Source: CAD feature listing. Evaluate the final solid. Frame: model axes, mm. A direction names the side the tool comes from. Round coordinates to 2 decimals unless told otherwise and drop trailing zeros. Write each loop counter-clockwise with the first axis right and the second up, starting at its lowest first coordinate (ties: lowest second). Pieces come first, ordered by that corner, then holes. Notation, with made-up numbers: (52, -32.75) -> (104, -32.75) arc R19 ccw to (104, -28.75) -> close; hole circle Ø11 at (35.5, 17). An arc over 180 degrees is marked (long way). Return JSON: item names as keys, results as strings. Group by question number.
from build123d import *

# Parameters (mm, degrees)
F1_DEPTH = 25
F2_R     = 14.710465
F3_DEPTH = 123


with BuildPart() as f1:
    # F0 (on Front) → F1 (new body)
    with BuildSketch(Plane.XZ):
        with BuildLine():
            ThreePointArc((34.69864, -4.583055), (34.924579, -2.296476), (35, 0))
            ThreePointArc((35, 0), (34.99986, 0.099012), (34.99944, 0.198024))
            ThreePointArc((34.99944, 0.198024), (34.930935, 2.197668), (34.748278, 4.190131))
            ThreePointArc((34.748278, 4.190131), (34.380054, 6.558346), (33.850622, 8.895809))
            ThreePointArc((33.850622, 8.895809), (33.286978, 10.815595), (32.614554, 12.700035))
            ThreePointArc((32.614554, 12.700035), (31.668947, 14.902275), (30.574844, 17.034638))
            ThreePointArc((30.574844, 17.034638), (29.551477, 18.753938), (28.431537, 20.41195))
            ThreePointArc((28.431537, 20.41195), (26.967963, 22.30984), (25.377937, 24.103118))
            ThreePointArc((25.377937, 24.103118), (23.959149, 25.513902), (22.462062, 26.841307))
            ThreePointArc((22.462062, 26.841307), (20.572484, 28.315595), (18.586441, 29.657111))
            ThreePointArc((18.586441, 29.657111), (16.861379, 30.670734), (15.081214, 31.584126))
            ThreePointArc((15.081214, 31.584126), (12.884359, 32.542177), (10.62709, 33.347638))
            ThreePointArc((10.62709, 33.347638), (8.704146, 33.900411), (6.752757, 34.342398))
            ThreePointArc((6.752757, 34.342398), (4.386663, 34.724015), (2, 34.94281))
            ThreePointArc((2, 34.94281), (0, 35), (-2, 34.94281))
            ThreePointArc((-2, 34.94281), (-4.386663, 34.724015), (-6.752757, 34.342398))
            ThreePointArc((-6.752757, 34.342398), (-8.704146, 33.900411), (-10.62709, 33.347638))
            ThreePointArc((-10.62709, 33.347638), (-12.884359, 32.542177), (-15.081214, 31.584126))
            ThreePointArc((-15.081214, 31.584126), (-16.861379, 30.670734), (-18.586441, 29.657111))
            ThreePointArc((-18.586441, 29.657111), (-20.572484, 28.315595), (-22.462062, 26.841307))
            ThreePointArc((-22.462062, 26.841307), (-23.959149, 25.513902), (-25.377937, 24.103118))
            ThreePointArc((-25.377937, 24.103118), (-26.967963, 22.30984), (-28.431537, 20.41195))
            ThreePointArc((-28.431537, 20.41195), (-29.551477, 18.753938), (-30.574844, 17.034638))
            ThreePointArc((-30.574844, 17.034638), (-31.668947, 14.902275), (-32.614554, 12.700035))
            ThreePointArc((-32.614554, 12.700035), (-33.286978, 10.815595), (-33.850622, 8.895809))
            ThreePointArc((-33.850622, 8.895809), (-34.380054, 6.558346), (-34.748278, 4.190131))
            ThreePointArc((-34.748278, 4.190131), (-34.930935, 2.197668), (-34.99944, 0.198024))
            ThreePointArc((-34.99944, 0.198024), (-34.930935, -2.197668), (-34.69864, -4.583055))
            ThreePointArc((-34.69864, -4.583055), (-34.380054, -6.558346), (-33.949115, -8.512204))
            ThreePointArc((-33.949115, -8.512204), (-33.286978, -10.815595), (-32.468759, -13.068271))
            ThreePointArc((-32.468759, -13.068271), (-31.668947, -14.902275), (-30.765642, -16.687579))
            ThreePointArc((-30.765642, -16.687579), (-29.551477, -18.753938), (-28.198746, -20.732359))
            ThreePointArc((-28.198746, -20.732359), (-26.967963, -22.30984), (-25.64905, -23.814412))
            ThreePointArc((-25.64905, -23.814412), (-23.959149, -25.513902), (-22.156903, -27.093757))
            ThreePointArc((-22.156903, -27.093757), (-20.572484, -28.315595), (-18.920835, -29.444898))
            ThreePointArc((-18.920835, -29.444898), (-16.861379, -30.670734), (-14.722859, -31.752754))
            ThreePointArc((-14.722859, -31.752754), (-12.884359, -32.542177), (-11.003753, -33.225253))
            ThreePointArc((-11.003753, -33.225253), (-8.704146, -33.900411), (-6.363725, -34.416609))
            ThreePointArc((-6.363725, -34.416609), (-4.386663, -34.724015), (-2.395266, -34.917942))
            ThreePointArc((-2.395266, -34.917942), (0, -35), (2.395266, -34.917942))
            ThreePointArc((2.395266, -34.917942), (4.386663, -34.724015), (6.363725, -34.416609))
            ThreePointArc((6.363725, -34.416609), (8.704146, -33.900411), (11.003753, -33.225253))
            ThreePointArc((11.003753, -33.225253), (12.884359, -32.542177), (14.722859, -31.752754))
            ThreePointArc((14.722859, -31.752754), (16.861379, -30.670734), (18.920835, -29.444898))
            ThreePointArc((18.920835, -29.444898), (20.572484, -28.315595), (22.156903, -27.093757))
            ThreePointArc((22.156903, -27.093757), (23.959149, -25.513902), (25.64905, -23.814412))
            ThreePointArc((25.64905, -23.814412), (26.967963, -22.30984), (28.198746, -20.732359))
            ThreePointArc((28.198746, -20.732359), (29.551477, -18.753938), (30.765642, -16.687579))
            ThreePointArc((30.765642, -16.687579), (31.668947, -14.902275), (32.468759, -13.068271))
            ThreePointArc((32.468759, -13.068271), (33.286978, -10.815595), (33.949115, -8.512204))
            ThreePointArc((33.949115, -8.512204), (34.380054, -6.558346), (34.69864, -4.583055))
        make_face()
        with BuildLine():
            ThreePointArc((34.748278, 4.190131), (34.930935, 2.197668), (34.99944, 0.198024))
            Line((34.99944, 0.198024), (39.921069, 2.511621))
            Line((39.921069, 2.511621), (34.748278, 4.190131))
        make_face()
        with BuildLine():
            Line((39.29149, -7.495253), (34.69864, -4.583055))
            ThreePointArc((34.69864, -4.583055), (34.380054, -6.558346), (33.949115, -8.512204))
            Line((33.949115, -8.512204), (39.29149, -7.495253))
        make_face()
        with BuildLine():
            ThreePointArc((32.614554, 12.700035), (33.286978, 10.815595), (33.850622, 8.895809))
            Line((33.850622, 8.895809), (38.042261, 12.36068))
            Line((38.042261, 12.36068), (32.614554, 12.700035))
        make_face()
        with BuildLine():
            Line((36.193082, -17.031172), (32.468759, -13.068271))
            ThreePointArc((32.468759, -13.068271), (31.668947, -14.902275), (30.765642, -16.687579))
            Line((30.765642, -16.687579), (36.193082, -17.031172))
        make_face()
        with BuildLine():
            ThreePointArc((28.431537, 20.41195), (29.551477, 18.753938), (30.574844, 17.034638))
            Line((30.574844, 17.034638), (33.773117, 21.433072))
            Line((33.773117, 21.433072), (28.431537, 20.41195))
        make_face()
        with BuildLine():
            Line((30.82053, -25.49696), (28.198746, -20.732359))
            ThreePointArc((28.198746, -20.732359), (26.967963, -22.30984), (25.64905, -23.814412))
            Line((25.64905, -23.814412), (30.82053, -25.49696))
        make_face()
        with BuildLine():
            ThreePointArc((22.462062, 26.841307), (23.959149, 25.513902), (25.377937, 24.103118))
            Line((25.377937, 24.103118), (27.381884, 29.158745))
            Line((27.381884, 29.158745), (22.462062, 26.841307))
        make_face()
        with BuildLine():
            Line((23.51141, -32.36068), (22.156903, -27.093757))
            ThreePointArc((22.156903, -27.093757), (20.572484, -28.315595), (18.920835, -29.444898))
            Line((18.920835, -29.444898), (23.51141, -32.36068))
        make_face()
        with BuildLine():
            ThreePointArc((15.081214, 31.584126), (16.861379, 30.670734), (18.586441, 29.657111))
            Line((18.586441, 29.657111), (19.270147, 35.052267))
            Line((19.270147, 35.052267), (15.081214, 31.584126))
        make_face()
        with BuildLine():
            Line((14.724982, -37.191059), (14.722859, -31.752754))
            ThreePointArc((14.722859, -31.752754), (12.884359, -32.542177), (11.003753, -33.225253))
            Line((11.003753, -33.225253), (14.724982, -37.191059))
        make_face()
        with BuildLine():
            ThreePointArc((6.752757, 34.342398), (8.704146, 33.900411), (10.62709, 33.347638))
            Line((10.62709, 33.347638), (9.947595, 38.743326))
            Line((9.947595, 38.743326), (6.752757, 34.342398))
        make_face()
        with BuildLine():
            Line((5.013329, -39.684588), (6.363725, -34.416609))
            ThreePointArc((6.363725, -34.416609), (4.386663, -34.724015), (2.395266, -34.917942))
            Line((2.395266, -34.917942), (5.013329, -39.684588))
        make_face()
        with BuildLine():
            ThreePointArc((-2, 34.94281), (0, 35), (2, 34.94281))
            Line((2, 34.94281), (0, 40))
            Line((0, 40), (-2, 34.94281))
        make_face()
        with BuildLine():
            Line((-5.013329, -39.684588), (-2.395266, -34.917942))
            ThreePointArc((-2.395266, -34.917942), (-4.386663, -34.724015), (-6.363725, -34.416609))
            Line((-6.363725, -34.416609), (-5.013329, -39.684588))
        make_face()
        with BuildLine():
            ThreePointArc((-10.62709, 33.347638), (-8.704146, 33.900411), (-6.752757, 34.342398))
            Line((-6.752757, 34.342398), (-9.947595, 38.743326))
            Line((-9.947595, 38.743326), (-10.62709, 33.347638))
        make_face()
        with BuildLine():
            Line((-14.724982, -37.191059), (-11.003753, -33.225253))
            ThreePointArc((-11.003753, -33.225253), (-12.884359, -32.542177), (-14.722859, -31.752754))
            Line((-14.722859, -31.752754), (-14.724982, -37.191059))
        make_face()
        with BuildLine():
            ThreePointArc((-18.586441, 29.657111), (-16.861379, 30.670734), (-15.081214, 31.584126))
            Line((-15.081214, 31.584126), (-19.270147, 35.052267))
            Line((-19.270147, 35.052267), (-18.586441, 29.657111))
        make_face()
        with BuildLine():
            Line((-23.51141, -32.36068), (-18.920835, -29.444898))
            ThreePointArc((-18.920835, -29.444898), (-20.572484, -28.315595), (-22.156903, -27.093757))
            Line((-22.156903, -27.093757), (-23.51141, -32.36068))
        make_face()
        with BuildLine():
            ThreePointArc((-25.377937, 24.103118), (-23.959149, 25.513902), (-22.462062, 26.841307))
            Line((-22.462062, 26.841307), (-27.381884, 29.158745))
            Line((-27.381884, 29.158745), (-25.377937, 24.103118))
        make_face()
        with BuildLine():
            Line((-30.82053, -25.49696), (-25.64905, -23.814412))
            ThreePointArc((-25.64905, -23.814412), (-26.967963, -22.30984), (-28.198746, -20.732359))
            Line((-28.198746, -20.732359), (-30.82053, -25.49696))
        make_face()
        with BuildLine():
            ThreePointArc((-30.574844, 17.034638), (-29.551477, 18.753938), (-28.431537, 20.41195))
            Line((-28.431537, 20.41195), (-33.773117, 21.433072))
            Line((-33.773117, 21.433072), (-30.574844, 17.034638))
        make_face()
        with BuildLine():
            Line((-36.193082, -17.031172), (-30.765642, -16.687579))
            ThreePointArc((-30.765642, -16.687579), (-31.668947, -14.902275), (-32.468759, -13.068271))
            Line((-32.468759, -13.068271), (-36.193082, -17.031172))
        make_face()
        with BuildLine():
            ThreePointArc((-33.850622, 8.895809), (-33.286978, 10.815595), (-32.614554, 12.700035))
            Line((-32.614554, 12.700035), (-38.042261, 12.36068))
            Line((-38.042261, 12.36068), (-33.850622, 8.895809))
        make_face()
        with BuildLine():
            Line((-39.29149, -7.495253), (-33.949115, -8.512204))
            ThreePointArc((-33.949115, -8.512204), (-34.380054, -6.558346), (-34.69864, -4.583055))
            Line((-34.69864, -4.583055), (-39.29149, -7.495253))
        make_face()
        with BuildLine():
            ThreePointArc((-34.99944, 0.198024), (-34.930935, 2.197668), (-34.748278, 4.190131))
            Line((-34.748278, 4.190131), (-39.921069, 2.511621))
            Line((-39.921069, 2.511621), (-34.99944, 0.198024))
        make_face()
    extrude(amount=F1_DEPTH)

    # F2 (on face) → F3 (cut)
    with BuildSketch(Plane.XZ.offset(25)):
        Circle(F2_R)
    extrude(amount=-F3_DEPTH, mode=Mode.SUBTRACT)


solid = f1.part
Item 1: First-contact query: pin 1 Ø2.5 at (y, z) = (-12.5, -33) entering from -X; pin 2 Ø2.5 at (y, z) = (-17.5, -35) entering from +X; pin 3 Ø4 at (x, y) = (-22, -13) entering from -Z. Flat tips, straight axial feed; report the tip coordinate or a pass-through.
Item 2: Cut plane B-B on x = 4. Output: boundary loops of the cut face in (y, z).
Item 3: Pull-direction query (X, two-part tool) for faces 5 (the flat face through (31.14, -12.32, 20.93)), 6 (the flat face through (22.844, -12.325, -29.764)), 7 (the cylindrical face through (-31.655, -12.325, 14.933)); classes: +X half, -X half, draft (parallel to the pull), parting line (faces both ways), or undercut.
Item 4: Set-up query: faces 1 (the flat face through (-34.305, -12.325, -15.022)), 2 (the cylindrical face through (-12.853, -12.325, 32.555)), 3 (the cylindrical face through (-8.7, -12.3, -33.9)), 4 (the cylindrical face through (-21, -12, 28)). Return all of +Z, -Z, +X, -X, +Y, -Y with unobstructed straight access to the full face (end or side cutting, diameter ignored); none if empty.
Item 5: Cut plane C-C on x = -17. Output: boundary loops of the cut face in (y, z).
Item 6: Cut plane A-A on z = -3. Output: boundary loops of the cut face in (x, y).
Item 7: Material intervals for probe 1 along X at (y, z) = (-17.5, 36); probe 2 along X at (y, z) = (-11, 29); probe 3 along Z at (x, y) = (36, -5.75), sorted ascending.
Here are the results:
{
 "1": {"pin 1": "stops at x = -23.51", "pin 2": "stops at x = 14.72", "pin 3": "stops at z = -32.36"},
 "2": {"outline": "(-25, -37.84) -> (0, -37.84) -> (0, -14.16) -> (-25, -14.16) -> close; (-25, 14.16) -> (0, 14.16) -> (0, 34.77) -> (-25, 34.77) -> close"},
 "3": {"face 5": "undercut", "face 6": "+X half", "face 7": "-X half"},
 "4": {"face 1": "-X, +Y, -Y", "face 2": "+Z, +Y, -Y", "face 3": "-Z, +Y, -Y", "face 4": "+Y, -Y"},
 "5": {"outline": "(-25, -30.59) -> (0, -30.59) -> (0, 33.17) -> (-25, 33.17) -> close"},
 "6": {"outline": "(-34.87, -25) -> (-14.4, -25) -> (-14.4, 0) -> (-34.87, 0) -> close; (14.4, -25) -> (34.87, -25) -> (34.87, 0) -> (14.4, 0) -> close"},
 "7": {"probe 1": "x = -10.29 to -7.96, -1.58 to 1.58, 7.96 to 10.29", "probe 2": "x = -27.32 to -27.04, -19.6 to 19.6, 27.04 to 27.32", "probe 3": "z = -17.02 to -16.83, -8.12 to -5.41, 0.67 to 3.78, 10.67 to 12.49"}
}
